Geometry: final body of the model. Coordinates: model frame, mm. A direction names the side the tool comes from. Coordinates: 2 decimals unless noted, no trailing zeros. Loops run counter-clockwise (first coordinate to the right, second up) from the corner with the lowest first, then second, coordinate; pieces in that order, holes last. Notation, with made-up numbers: (58, 55.5) - (81, 55.5) arc R16 cw to (81, 76.5) - close; hole circle Ø1 at (-11, 44). An arc over 180 degrees is marked (long way). Return JSON: item names as keys, results as strings.
from build123d import *

# Parameters (mm, degrees)
SKETCH1_W           = 40
SKETCH1_H           = 30
BOSS_EXTRUDE1_DEPTH = 8
SKETCH4_R           = 1.45
SKETCH4_W           = 34
SKETCH4_H           = 20
CUT_EXTRUDE1_DEPTH  = 5
SKETCH5_R           = 2.975
BOSS_EXTRUDE2_DEPTH = 5


with BuildPart() as part:
    # Sketch1 → Boss-Extrude1 (new body)
    with BuildSketch(Plane(origin=(0, 0, 0), x_dir=(0, 0, -1), z_dir=(1, 0, 0))):
        with Locations((20, 15)):
            Rectangle(SKETCH1_W, SKETCH1_H)
    extrude(amount=BOSS_EXTRUDE1_DEPTH)

    # Sketch4 → Cut-Extrude1 (cut)
    with BuildSketch(Plane(origin=(8, 0, 0), x_dir=(0, 0, -1), z_dir=(1, 0, 0))):
        with Locations((37, 27)):
            Circle(SKETCH4_R)
        with Locations((3, 27)):
            Circle(SKETCH4_R)
        with Locations((3, 3)):
            Circle(SKETCH4_R)
        with Locations((37, 3)):
            Circle(SKETCH4_R)
        with Locations((20, 15)):
            Rectangle(SKETCH4_W, SKETCH4_H)
    extrude(amount=-CUT_EXTRUDE1_DEPTH, mode=Mode.SUBTRACT)

    # Sketch5 → Boss-Extrude2 (add)
    with BuildSketch(Plane(origin=(3, 0, 0), x_dir=(0, 0, -1), z_dir=(1, 0, 0))):
        with Locations(Location((8.5, 17, 0), (0, 0, 180))):
            Circle(SKETCH5_R)
        with Locations(Location((20, 15, 0), (0, 0, 180))):
            Circle(SKETCH5_R)
        with Locations(Location((31.5, 17, 0), (0, 0, 180))):
            Circle(SKETCH5_R)
    extrude(amount=BOSS_EXTRUDE2_DEPTH)


solid = part.part
Item 1: Section query C-C, the plane z = -8.5. Return loops of the section in (x, y) (3 decimals), and give its area (3 significant figures).
Worked out:
{"outline": "(0, 0) - (8, 0) - (8, 5) - (3, 5) - (3, 14.025) - (8, 14.025) - (8, 19.975) - (3, 19.975) - (3, 25) - (8, 25) - (8, 30) - (0, 30) - close", "area": "170 mm^2"}
Item 2: Mould query, pull axis Z, two halves, no side actions, for faces 1 (the face through (5.54, 3.06, -1.55)), 2 (the face through (4, 0, -20)), 3 (the face through (4, 15, 0)). Classes: +Z half, -Z half, draft (parallel to the pull), parting line (faces both ways), or undercut.
Worked out:
{"face 1": "undercut", "face 2": "draft", "face 3": "+Z half"}
Item 3: Section query B-B, the plane y = 3. Return loops of the section in (x, z), and give its area (3 significant figures).
Worked out:
{"outline": "(0, -40) - (8, -40) - (8, -38.45) - (3, -38.45) - (3, -35.55) - (8, -35.55) - (8, -4.45) - (3, -4.45) - (3, -1.55) - (8, -1.55) - (8, 0) - (0, 0) - close", "area": "291 mm^2"}
Item 4: Reachability of faces 4 (the face through (4, 30, -20)), 5 (the face through (3, 27, -3)) from +Z, -Z, +X, -X, +Y, -Y: full face, straight path, thin tool, end or side. Return the list, or none.
Worked out:
{"face 4": "+Z, -Z, +X, -X, +Y", "face 5": "+X"}
Item 5: Section query A-A, the plane x = 7. Count the separate pieces of the cut face and the enclosed holes in it, and give its area (3 significant figures).
Worked out:
{"separate pieces": "4", "enclosed holes": "5", "area": "577 mm^2"}
Item 6: Ray query, probe 1 along Y at (x, z) = (4.5, -7.5); probe 2 along Z at (x, y) = (7.5, 22.5); probe 3 along Y at (x, z) = (5.25, -19.5). Return the intervals inside material, ascending. Write a range as from..to.
Worked out:
{"probe 1": "0..5, 14.2..19.8, 25..30", "probe 2": "-40..-37, -3..0", "probe 3": "0..5, 12.07..17.93, 25..30"}
Item 7: Section query D-D, the plane y = 10.5. Return loops of the section in (x, z).
Worked out:
{"outline": "(0, -40) - (8, -40) - (8, -37) - (3, -37) - (3, -3) - (8, -3) - (8, 0) - (0, 0) - close"}
Item 8: First-contact query: pin 1 Ø0.9 at (y, z) = (2.5, -37) entering from +X. Flat tip, straight axial feed; report the tip coordinate or a pass-through.
Worked out:
{"pin 1": "x = 3"}
